from build123d import *

# Parameters (mm, degrees)
SKIZZE1_W                       = 215
SKIZZE1_H                       = 87
AUFSATZ_LINEAR_AUSTRAGEN1_DEPTH = 145
WANDUNG1_T                      = 3


with BuildPart() as part:
    # Skizze1 → Aufsatz-Linear austragen1 (new, symmetric)
    with BuildSketch(Plane.XY):
        Rectangle(SKIZZE1_W, SKIZZE1_H)
    extrude(amount=AUFSATZ_LINEAR_AUSTRAGEN1_DEPTH, both=True)

    # Wandung1
    wandung1_openings = [part.faces().sort_by_distance(p)[0] for p in [
        (0, 43.5, 0),
    ]]
    offset(amount=WANDUNG1_T, openings=wandung1_openings, kind=Kind.INTERSECTION)


solid = part.part
Work out the finished part from the listing and answer in its coordinate system (mm). A direction names the side the tool comes from. Coordinates: 2 decimals unless noted, no trailing zeros. Write each loop counter-clockwise with the first axis right and the second up, starting at its lowest first coordinate (ties: lowest second). Pieces come first, ordered by that corner, then holes. Notation, with made-up numbers: M 42,51 L 86,51 A14 ccw 86,68 Z; hole C 56.5,70 d2. An arc over 180 degrees is marked long. Write item = value, one per line.
1. A flat-ended cylindrical pin translates along its axis: pin 1 (1.5 mm diameter, centred on x = -73.5, z = -34.5, fed in from +Y). Find the tip coordinate at first contact, or state that the pin passes through.
Solution:
pin_1 = -43.5
2. Straight lines are drawn through the part: line 1 (X direction, y = -4, z = 20.5); line 2 (Z direction, x = 101, y = 0); line 3 (Y direction, x = -61, z = -42). For each, find the intervals that lie inside material, in ascending order. Write a range as from..to.
Solution:
line_1 = -110.5..-107.5, 107.5..110.5
line_2 = -148..-145, 145..148
line_3 = -46.5..-43.5
3. Determine the mould class of faces 1 (the face through (-107.5, -1, 2)), 2 (the face through (-2, -46.5, 2)), 3 (the face through (110.5, -2, 2)) for opening direction X: released by +X, released by -X, zero draft, split by the parting line, or undercut.
Solution:
face_1 = undercut
face_2 = zero draft
face_3 = released by +X
4. The part is cut by section B-B (z = -111). Determine the outline of the cut face in (x, y), then the cut area to 4 significant figures.
Solution:
outline = M -110.5,-46.5 L 110.5,-46.5 L 110.5,43.5 L 107.5,43.5 L 107.5,-43.5 L -107.5,-43.5 L -107.5,43.5 L -110.5,43.5 Z
area = 1,185 mm2
5. The part is cut by section A-A (y = 23.5). Determine the outline of the cut face in (x, z), then the cut area to 3 significant figures.
Solution:
outline = M -110.5,-148 L 110.5,-148 L 110.5,148 L -110.5,148 Z; hole M -107.5,-145 L 107.5,-145 L 107.5,145 L -107.5,145 Z
area = 3,070 mm2
6. The part is cut by section C-C (x = 42). Determine the outline of the cut face in (y, z).
Solution:
outline = M -46.5,-148 L 43.5,-148 L 43.5,-145 L -43.5,-145 L -43.5,145 L 43.5,145 L 43.5,148 L -46.5,148 Z
7. For faces 4 (the face through (-2, -1, -148)), 5 (the face through (107.5, -1, 2)), determine the directions among +Z, -Z, +X, -X, +Y, -Y from which every point of the face is accessible in a straight line to the end or side of a thin tool.
Solution:
face_4 = -Z, +X, -X, +Y, -Y
face_5 = +Y
